Print and shaded views of the part. All mm, measured from the part's lowest x, y and z. A direction names the side the tool comes from. Coordinates: 2 decimals unless noted, no trailing zeros. Order: outer loops, then holes, each group sorted by start corner. A loop starts at its lowest first (then second) coordinate and runs counter-clockwise, first axis right, second up. Notation, with made-up numbers: (2.5, 83) -> (38.5, 83) arc R27 cw to (38.5, 114) -> close; hole circle Ø6 at (66.5, -7). An arc over 180 degrees is marked (long way). Use one line per item in the form item = value. Start each with the question number.
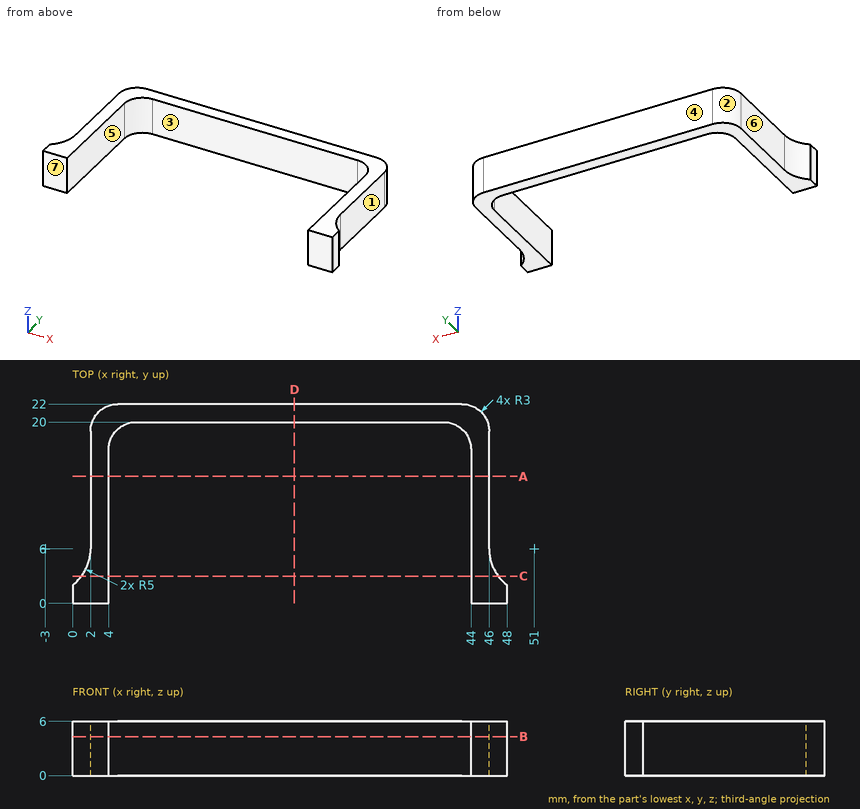
1) Cut at C-C on y = 3. Give the cut face in (x, z), then the cut area to 3 significant figures.
2) Cut at D-D on x = 24.5. Give the cut face in (y, z), then the cut area to 3 significant figures.
3) Probe L1, parallel to X at y = 9, z = 2.9; L2, parallel to Y at x = 16.5, z = 3.5; L3, parallel to X at y = 19.5, z = 3.55. List the from-to ranges inside material, lowest first.
4) Two-plate mould, pull along X, no slides. Class the marked faces 1, 2, 3 and 4: released by +X, released by -X, zero draft, split by the parting line, or undercut.
5) Cut at A-A on y = 14. Give the cut face in (x, z).
6) 3-axis set-ups, long thin cutter, end or side, ignore diameter. For the marked faces 5, 6 and 7: which of +Z, -Z, +X, -X, +Y, -Y reach the whole face in a straight line?
7) Drop flat-ended pins along their axis: P1, Ø1.8, axis at y = 10.5, z = 3.5, coming from the +X side; P2, Ø1, axis at x = 15.5, z = 3, coming from the -Y side; P3, Ø10, axis at x = 12, y = 17, coming from the +Z side; P4, Ø3, axis at y = 15.5, z = 3, coming from the -X side. Give the stop position or say it passes through.
8) Cut at B-B on z = 4.3. Give the cut face in (x, y), then the cut area to 3 significant figures.
Values follow:
q1.outline = (1, 0) -> (4, 0) -> (4, 6) -> (1, 6) -> close; (44, 0) -> (47, 0) -> (47, 6) -> (44, 6) -> close
q1.area = 36.0 mm^2
q2.outline = (20, 0) -> (22, 0) -> (22, 6) -> (20, 6) -> close
q2.area = 12.0 mm^2
q3.L1 = 2 to 4, 44 to 46
q3.L2 = 20 to 22
q3.L3 = 2.04 to 5.34, 42.66 to 45.96
q4.face_1 = released by +X
q4.face_2 = released by -X
q4.face_3 = undercut
q4.face_4 = zero draft
q5.outline = (2, 0) -> (4, 0) -> (4, 6) -> (2, 6) -> close; (44, 0) -> (46, 0) -> (46, 6) -> (44, 6) -> close
q6.face_5 = +Z, -Z, -Y
q6.face_6 = +Z, -Z, -X, +Y
q6.face_7 = +Z, -Z, +X, -X, -Y
q7.P1 = 46
q7.P2 = 20
q7.P3 = 6
q7.P4 = 2
q8.outline = (0, 0) -> (4, 0) -> (4, 17) arc R3 cw to (7, 20) -> (41, 20) arc R3 cw to (44, 17) -> (44, 0) -> (48, 0) -> (48, 2) arc R5 cw to (46, 6) -> (46, 19) arc R3 ccw to (43, 22) -> (5, 22) arc R3 ccw to (2, 19) -> (2, 6) arc R5 cw to (0, 2) -> close
q8.area = 181 mm^2
